```python
from build123d import *

# Parameters (mm, degrees)
SKETCH1_R           = 3.8
SKETCH1_R_2         = 2.15
BOSS_EXTRUDE1_DEPTH = 35.7
CUT_EXTRUDE1_DEPTH  = 0.3


with BuildPart() as part:
    # Sketch1 → Boss-Extrude1 (new body)
    with BuildSketch(Plane(origin=(0, 0, 0), x_dir=(1, 0, 0), z_dir=(0, 1, 0))):
        with Locations(Location((0, 0, 0), (0, 0, 90))):
            Circle(SKETCH1_R)
        with Locations(Location((0, 0, 0), (0, 0, 90))):
            Circle(SKETCH1_R_2, mode=Mode.SUBTRACT)
    extrude(amount=BOSS_EXTRUDE1_DEPTH)

    # Sketch2 → Cut-Extrude1 (cut)
    # profile 1 of 4: a face of its own
    with BuildSketch(Plane(origin=(0, 35.7, 0), x_dir=(1, 0, 0), z_dir=(0, 1, 0))):
        with BuildLine():
            Line((2.111656105, -0.681757882), (2.144411013, -0.370109244))
            add(Edge.make_bspline(
                [(2.144411013, -0.370109244), (2.146802183, -0.348691162), (2.15138598, -0.307633396), (2.158693119, -0.248902879), (2.165911145, -0.195653849), (2.173439795, -0.148026639), (2.181405599, -0.105945418), (2.189365932, -0.069370665), (2.196899512, -0.038121368), (2.203230185, -0.019522424), (2.206104723, -0.011077293)],
                knots=[0, 0, 0, 0, 1.417373572, 2.717059047, 3.892315439, 4.951364628, 5.887982497, 6.708448809, 7.413551636, 8, 8, 8, 8], degree=3))
            add(Edge.make_bspline(
                [(2.206104723, -0.011077293), (2.210142486, -0.000387677), (2.218120236, 0.020732699), (2.233480051, 0.050530823), (2.249714506, 0.079217068), (2.26903293, 0.105377158), (2.28975844, 0.130224476), (2.312780938, 0.153046655), (2.337556691, 0.174424753), (2.364307409, 0.193873427), (2.392778115, 0.210986132), (2.422871362, 0.225484332), (2.454400246, 0.23669106), (2.487041624, 0.245969514), (2.521307609, 0.251371473), (2.556788909, 0.254755049), (2.593708427, 0.254583895), (2.61857229, 0.252608033), (2.631282507, 0.251597988)],
                knots=[0, 0, 0, 0, 1.011284266, 1.998079665, 2.96593116, 3.927568455, 4.873724646, 5.829799179, 6.795279379, 7.770029274, 8.755528345, 9.734069651, 10.723185245, 11.716348137, 12.735145537, 13.790957307, 14.870754256, 16, 16, 16, 16], degree=3))
            add(Edge.make_bspline(
                [(2.631282507, 0.251597988), (2.644032058, 0.24997818), (2.668933898, 0.246814446), (2.705191942, 0.239067164), (2.739499602, 0.22904372), (2.771695562, 0.216250901), (2.801935318, 0.201182094), (2.830167738, 0.18375954), (2.856506904, 0.163892672), (2.880584442, 0.141642816), (2.902598289, 0.117288438), (2.922659945, 0.091347366), (2.940268337, 0.063416255), (2.955457965, 0.033787663), (2.968650724, 0.002594273), (2.978949316, -0.030497322), (2.987853849, -0.065140381), (2.991380402, -0.089158794), (2.993176538, -0.101391796)],
                knots=[0, 0, 0, 0, 1.120443029, 2.188398027, 3.229732507, 4.234008471, 5.205583901, 6.172795254, 7.123159449, 8.078367438, 9.027336717, 9.98330492, 10.934837467, 11.902358037, 12.884432561, 13.884316223, 14.922444945, 16, 16, 16, 16], degree=3))
            add(Edge.make_bspline(
                [(2.993176538, -0.101391796), (2.994230251, -0.111454082), (2.996521933, -0.133338158), (2.997952687, -0.169220751), (2.997758266, -0.210688547), (2.99653436, -0.257987318), (2.99350795, -0.310882297), (2.989330268, -0.36950307), (2.984003426, -0.433765073), (2.979373477, -0.478452172), (2.976958088, -0.501764893)],
                knots=[0, 0, 0, 0, 0.604865624, 1.315498741, 2.145858656, 3.084317767, 4.144404289, 5.313618666, 6.59854729, 8, 8, 8, 8], degree=3))
            Line((2.976958088, -0.501764893), (2.965191762, -0.613385986))
            Line((2.965191762, -0.613385986), (3.69247792, -0.689708102))
            Line((3.69247792, -0.689708102), (3.675941462, -0.846168438))
            Line((3.675941462, -0.846168438), (2.111656105, -0.681757882))
        make_face()
        with BuildLine():
            Line((2.280200776, -0.541515995), (2.811911514, -0.597167537))
            Line((2.811911514, -0.597167537), (2.843076377, -0.332902212))
            add(Edge.make_bspline(
                [(2.843076377, -0.332902212), (2.844289329, -0.319974038), (2.846633891, -0.294984657), (2.849267306, -0.258732107), (2.850574992, -0.225003014), (2.8506223, -0.193920252), (2.849446171, -0.165468856), (2.846833591, -0.139695973), (2.843533978, -0.116385305), (2.837224352, -0.089138127), (2.826277417, -0.05801598), (2.808152361, -0.023948438), (2.784508643, 0.006287227), (2.756461903, 0.032531622), (2.725026024, 0.054952555), (2.690476942, 0.072174184), (2.653338622, 0.084201266), (2.627543305, 0.088078292), (2.61442804, 0.09004951)],
                knots=[0, 0, 0, 0, 1.137510035, 2.198738341, 3.183774331, 4.093820263, 4.921124839, 5.676965373, 6.362509616, 6.981975284, 8.12447774, 9.242103714, 10.347315548, 11.470636665, 12.59656481, 13.717849775, 14.83967295, 16, 16, 16, 16], degree=3))
            add(Edge.make_bspline(
                [(2.61442804, 0.09004951), (2.601492156, 0.090867689), (2.575975574, 0.092481581), (2.537925492, 0.088020007), (2.500904783, 0.078506725), (2.46570153, 0.063177958), (2.43299178, 0.043746262), (2.404191117, 0.019855084), (2.379800983, -0.008048068), (2.363216589, -0.034756124), (2.351731956, -0.058692023), (2.344337638, -0.079917763), (2.337050019, -0.103790363), (2.329926737, -0.130456035), (2.324165305, -0.160160444), (2.318330265, -0.192568564), (2.313285026, -0.227894023), (2.310555246, -0.252437869), (2.309139579, -0.265166335)],
                knots=[0, 0, 0, 0, 1.162655522, 2.293387438, 3.425402363, 4.586027317, 5.731110208, 6.83356732, 7.933882776, 9.046497222, 9.647242429, 10.316155155, 11.063354823, 11.890427355, 12.794535371, 13.781081296, 14.849266247, 16, 16, 16, 16], degree=3))
            Line((2.309139579, -0.265166335), (2.280200776, -0.541515995))
        make_face(mode=Mode.SUBTRACT)
    # profile 2 of 4: a face of its own
    with BuildSketch(Plane(origin=(0, 35.7, 0), x_dir=(1, 0, 0), z_dir=(0, 1, 0))):
        Polygon((2.170881214, 0.473456425), (2.136218253, 0.627054682), (3.671246799, 0.973366281), (3.705909759, 0.819768024), align=None)
    # profile 3 of 4: a face of its own
    with BuildSketch(Plane(origin=(0, 35.7, 0), x_dir=(1, 0, 0), z_dir=(0, 1, 0))):
        with BuildLine():
            Line((-2.056988676, 0.799308725), (-2.108188095, 0.487660087))
            add(Edge.make_bspline(
                [(-2.108188095, 0.487660087), (-2.111708879, 0.466232817), (-2.118445766, 0.425232539), (-2.129421133, 0.36665679), (-2.139718713, 0.313480105), (-2.150281282, 0.265914926), (-2.160212249, 0.223828754), (-2.170557002, 0.187532109), (-2.179974067, 0.156559724), (-2.187465233, 0.138231414), (-2.190870387, 0.129900171)],
                knots=[0, 0, 0, 0, 1.41672968, 2.710859107, 3.888203329, 4.950446671, 5.889832269, 6.708755629, 7.413057157, 8, 8, 8, 8], degree=3))
            add(Edge.make_bspline(
                [(-2.190870387, 0.129900171), (-2.195556444, 0.11941634), (-2.204838325, 0.098650549), (-2.221929721, 0.069508001), (-2.240455136, 0.041959041), (-2.260630824, 0.016005619), (-2.28356608, -0.007341147), (-2.307553717, -0.029678541), (-2.334263373, -0.049103372), (-2.362013715, -0.067435737), (-2.391696978, -0.083048929), (-2.422778873, -0.095769744), (-2.455093773, -0.105304128), (-2.488524604, -0.111948097), (-2.523172883, -0.116205202), (-2.559155273, -0.11708093), (-2.596246189, -0.114743131), (-2.621154486, -0.111310806), (-2.633856665, -0.109560466)],
                knots=[0, 0, 0, 0, 1.008565843, 1.997711397, 2.964088398, 3.925828959, 4.881231488, 5.837542023, 6.8027058, 7.77948986, 8.758803017, 9.744916733, 10.726487241, 11.714930589, 12.737596956, 13.790702482, 14.873351644, 16, 16, 16, 16], degree=3))
            add(Edge.make_bspline(
                [(-2.633856665, -0.109560466), (-2.646618171, -0.107204254), (-2.671598778, -0.102591978), (-2.707626521, -0.092636992), (-2.741459416, -0.080586731), (-2.773228531, -0.066238595), (-2.802791732, -0.049368652), (-2.830283852, -0.030242912), (-2.855627907, -0.008737139), (-2.878770231, 0.014985273), (-2.899399946, 0.040920795), (-2.917983767, 0.068252889), (-2.933935366, 0.097479257), (-2.94758708, 0.128207774), (-2.958694781, 0.160590944), (-2.967721239, 0.194453712), (-2.973992641, 0.230009053), (-2.976403376, 0.254328418), (-2.977624193, 0.266643961)],
                knots=[0, 0, 0, 0, 1.121688944, 2.195702573, 3.227831976, 4.224598539, 5.20573391, 6.166885501, 7.116340498, 8.07565474, 9.027584121, 9.978365483, 10.930074198, 11.902608988, 12.882373339, 13.887282389, 14.930101006, 16, 16, 16, 16], degree=3))
            add(Edge.make_bspline(
                [(-2.977624193, 0.266643961), (-2.978173535, 0.276817647), (-2.979369039, 0.2989581), (-2.978416522, 0.335055248), (-2.97575293, 0.376716727), (-2.971541929, 0.424106537), (-2.965863423, 0.477242518), (-2.958062562, 0.535941987), (-2.94893467, 0.60032135), (-2.941666402, 0.644981141), (-2.937873091, 0.668289093)],
                knots=[0, 0, 0, 0, 0.604646202, 1.315859532, 2.141770145, 3.082979908, 4.139987401, 5.313936572, 6.598143075, 8, 8, 8, 8], degree=3))
            Line((-2.937873091, 0.668289093), (-2.919746589, 0.779910187))
            Line((-2.919746589, 0.779910187), (-3.647032747, 0.898845483))
            Line((-3.647032747, 0.898845483), (-3.621274033, 1.05530582))
            Line((-3.621274033, 1.05530582), (-2.056988676, 0.799308725))
        make_face()
        with BuildLine():
            Line((-2.234755603, 0.667653076), (-2.766466341, 0.754787491))
            Line((-2.766466341, 0.754787491), (-2.812895628, 0.490840175))
            add(Edge.make_bspline(
                [(-2.812895628, 0.490840175), (-2.815008197, 0.477922044), (-2.81910293, 0.452883193), (-2.823415086, 0.416473146), (-2.826657363, 0.382653714), (-2.828734553, 0.35136981), (-2.829006368, 0.322605404), (-2.828117211, 0.296281893), (-2.825997962, 0.272585261), (-2.82146303, 0.244692822), (-2.811909992, 0.212873549), (-2.795853791, 0.177447593), (-2.773735167, 0.14572244), (-2.747345259, 0.117404003), (-2.716955042, 0.093039199), (-2.682766519, 0.074626688), (-2.646499979, 0.05943945), (-2.620631779, 0.054501823), (-2.607461934, 0.051988011)],
                knots=[0, 0, 0, 0, 1.136739534, 2.20331033, 3.183538476, 4.087470488, 4.925317766, 5.680760515, 6.37425325, 6.990267555, 8.132251804, 9.248525494, 10.354270943, 11.474675275, 12.601942906, 13.718823886, 14.838622839, 16, 16, 16, 16], degree=3))
            add(Edge.make_bspline(
                [(-2.607461934, 0.051988011), (-2.594553232, 0.050310074), (-2.568992641, 0.046987581), (-2.53033584, 0.049159746), (-2.492576023, 0.056899765), (-2.456092773, 0.069822513), (-2.422214957, 0.08795422), (-2.391742809, 0.110088649), (-2.365813449, 0.136873568), (-2.347514733, 0.162509328), (-2.334999931, 0.186178026), (-2.325732889, 0.206848206), (-2.317397434, 0.230587534), (-2.308596743, 0.25697407), (-2.300834458, 0.286429563), (-2.293637242, 0.318843854), (-2.286151391, 0.353972674), (-2.282041679, 0.378564756), (-2.279912855, 0.391303416)],
                knots=[0, 0, 0, 0, 1.158878903, 2.294702534, 3.43304114, 4.587206463, 5.733290821, 6.84883061, 7.931810954, 9.043940833, 9.644510014, 10.317362802, 11.062023369, 11.887125953, 12.797502392, 13.776738287, 14.848353887, 16, 16, 16, 16], degree=3))
            Line((-2.279912855, 0.391303416), (-2.234755603, 0.667653076))
        make_face(mode=Mode.SUBTRACT)
    # profile 4 of 4: a face of its own
    with BuildSketch(Plane(origin=(0, 35.7, 0), x_dir=(1, 0, 0), z_dir=(0, 1, 0))):
        Polygon((-2.194903236, -0.321716904), (-2.166600452, -0.476587196), (-3.716257403, -0.758343006), (-3.744560187, -0.603472713), align=None)
    extrude(amount=-CUT_EXTRUDE1_DEPTH, mode=Mode.SUBTRACT)


solid = part.part
```
Can you work these out from the model? Positions are in its coordinate system, mm. Give positions to 0.01 mm unless a question says otherwise; leave off trailing zeros. Loops run counter-clockwise (first coordinate to the right, second up) from the corner with the lowest first, then second, coordinate; pieces in that order, holes last. Notation, with made-up numbers: M -7.75,37.25 L 21.25,37.25 A10 cw 21.25,53.25 Z; hole C -39,21.5 d9. An arc over 180 degrees is marked long. One line per question, with ' | ' between items. Start each with the question number.
Q1. If we mould it in two halves opening along Z, with no side actions, what happens to faces 1 (the flat face through (2, 35.7, -2)), 2 (the cylindrical face through (1.308, 17.6, 1.706)), 3 (the cylindrical face through (1.46, 17.6, -3.51))? For each: +Z half, -Z half, draft (parallel to the pull), parting line (faces both ways), or undercut.
Q2. If I drill on line 1 (X direction, y = 17, z = 0); line 2 (Z direction, x = 0.5, y = 15.5); line 3 (Z direction, x = 1, y = 23), over which ranges is the centre line in solid material (lowest first)? Write a range as from..to.
Q3. If we section it at C-C (y = 12): Please give me the cut outline in (x, z), plus the area to 3 significant figures.
Q4. For pin 1 Ø1.5 at (y, z) = (11, 0.5) entering from +X; pin 2 Ø1 at (y, z) = (14.5, 1) entering from -X; pin 3 Ø1 at (y, z) = (6, 2.5) entering from +X; pin 4 Ø2 at (x, y) = (-2.5, 32) entering from +Z, each with a flat end and sliding along its axis, tell me the tip position at first contact or that it passes through.
Q5. If we section it at A-A (x = 0): Please give me the cut outline in (y, z).
Q6. If we section it at B-B (z = -1.75): Please give me the cut outline in (x, y), plus the area to 3 significant figures.
Computed:
1) face 1: draft | face 2: undercut | face 3: parting line
2) line 1: x = -3.8..-2.15, 2.15..3.8 | line 2: z = -3.77..-2.09, 2.09..3.77 | line 3: z = -3.67..-1.9, 1.9..3.67
3) outline: C 0,0 d7.6; hole C 0,0 d4.3 | area: 30.8 mm²
4) pin 1: stops at x = 3.8 | pin 2: stops at x = -3.77 | pin 3: stops at x = 3.23 | pin 4: stops at z = 3.49
5) outline: M 0,-3.8 L 35.7,-3.8 L 35.7,-2.15 L 0,-2.15 Z; M 0,2.15 L 35.7,2.15 L 35.7,3.8 L 0,3.8 Z
6) outline: M -3.37,0 L -1.25,0 L -1.25,35.7 L -3.37,35.7 Z; M 1.25,0 L 3.37,0 L 3.37,35.7 L 1.25,35.7 Z | area: 152 mm²
